The figure shows three views and two pictorial views of one solid part (mm, origin at its lowest corner). Answer the questions. A direction names the side the tool comes from. Coordinates: 2 decimals unless noted, no trailing zeros. Order: outer loops, then holes, each group sorted by start corner. A loop starts at its lowest first (then second) coordinate and runs counter-clockwise, first axis right, second up. Notation, with made-up numbers: M 15,-38 L 61,-38 A26 ccw 61,-7 Z; hole C 10.5,-6.75 d4. An arc over 180 degrees is marked long. Answer in a Markdown table with one row per item. Add a question column.
Item 1: The part is cut by section D-D (x = 9.25). Write down the section's boundary in (y, z).
Item 2: The mould has two halves that part along Y. Classify the marked faces 4, 5 and 6: released by +Y, released by -Y, zero draft, split by the parting line, or undercut.
Item 3: Which of the six approach directions +Z, -Z, +X, -X, +Y, -Y give full straight-line access (tool end or side, diameter ignored) to the marked faces 1, 2 and 3?
Item 4: The part is cut by section C-C (z = 0.75). Write down the section's boundary in (x, y).
Item 5: The part is cut by section A-A (y = 19.5). Write down the section's boundary in (x, z).
Item 6: Consider line 1 (Y direction, x = 5, z = 6.7); line 2 (Y direction, x = 9, z = 5.25); line 3 (X direction, y = 19.5, z = 6.7). Determine where each line is inside the solid, lowest interval first. Write a range as from..to.
Item 7: The part is cut by section B-B (x = 5). Write down the section's boundary in (y, z).
Item 8: Flat-ended cylindrical pins translate along their axes: pin 1 Ø5 at (x, y) = (5.5, 20) entering from -Z; pin 2 Ø3 at (x, y) = (4, 29.5) entering from +Z; pin 3 Ø5 at (x, y) = (2.5, 20) entering from -Z; pin 4 Ø3 at (x, y) = (5, 19.5) entering from -Z. Find the tip coordinate at first contact, or state that the pin passes through.
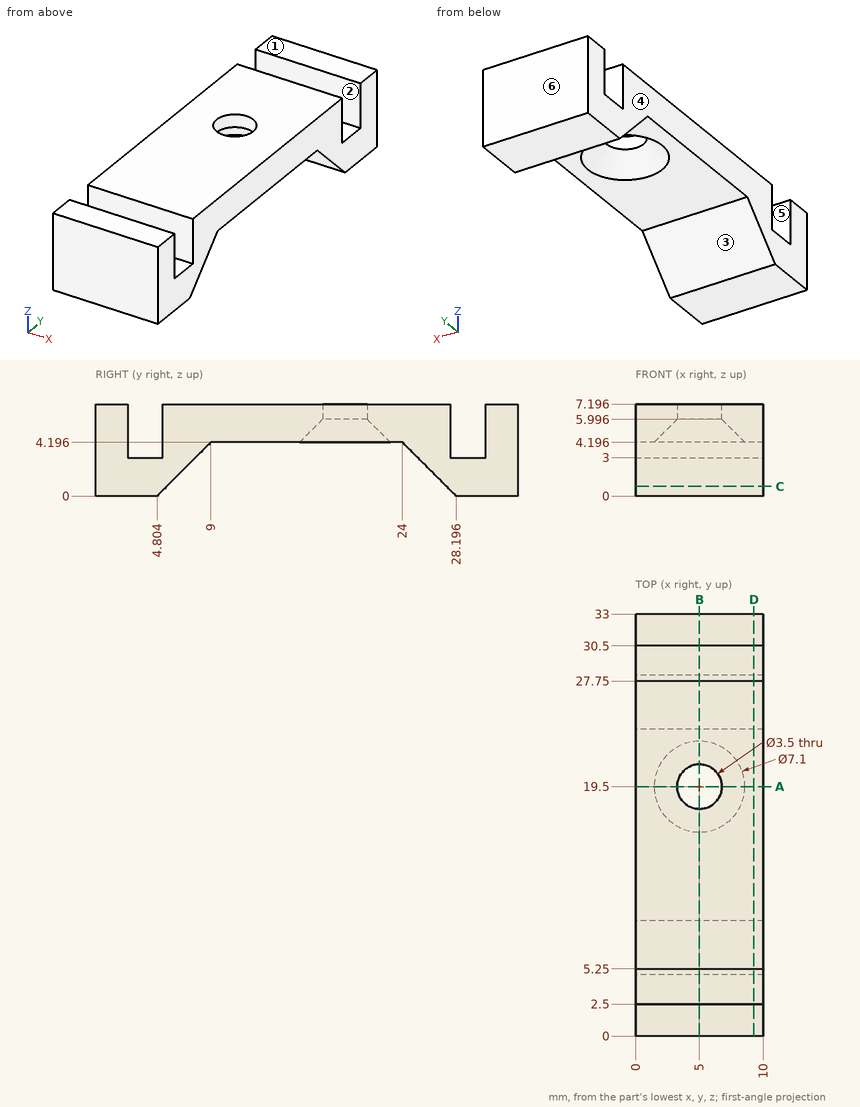
Reply:
| question | item | result |
|---|---|---|
| 1 | outline | M 0,0 L 4.8,0 L 9,4.2 L 24,4.2 L 28.2,0 L 33,0 L 33,7.2 L 30.5,7.2 L 30.5,3 L 27.75,3 L 27.75,7.2 L 5.25,7.2 L 5.25,3 L 2.5,3 L 2.5,7.2 L 0,7.2 Z |
| 2 | face 4 | zero draft |
| 2 | face 5 | undercut |
| 2 | face 6 | released by +Y |
| 3 | face 1 | +Z, +X, -X, +Y, -Y |
| 3 | face 2 | +Z, +X, -X |
| 3 | face 3 | -Z, +X, -X |
| 4 | outline | M 0,0 L 10,0 L 10,5.55 L 0,5.55 Z; M 0,27.45 L 10,27.45 L 10,33 L 0,33 Z |
| 5 | outline | M 0,4.2 L 1.45,4.2 L 3.25,6 L 3.25,7.2 L 0,7.2 Z; M 6.75,6 L 8.55,4.2 L 10,4.2 L 10,7.2 L 6.75,7.2 Z |
| 6 | line 1 | y = 0..2.5, 5.25..17.75, 21.25..27.75, 30.5..33 |
| 6 | line 2 | y = 0..2.5, 5.25..27.75, 30.5..33 |
| 6 | line 3 | x = 0..3.25, 6.75..10 |
| 7 | outline | M 0,0 L 4.8,0 L 9,4.2 L 15.95,4.2 L 17.75,6 L 17.75,7.2 L 5.25,7.2 L 5.25,3 L 2.5,3 L 2.5,7.2 L 0,7.2 Z; M 21.25,6 L 23.05,4.2 L 24,4.2 L 28.2,0 L 33,0 L 33,7.2 L 30.5,7.2 L 30.5,3 L 27.75,3 L 27.75,7.2 L 21.25,7.2 Z |
| 8 | pin 1 | stops at z = 4.54 |
| 8 | pin 2 | stops at z = 7.2 |
| 8 | pin 3 | stops at z = 4.2 |
| 8 | pin 4 | passes through |
